Geometry: final body of the model. Coordinates: model frame, mm. Give positions to 0.01 mm unless a question says otherwise; leave off trailing zeros. Write each loop counter-clockwise with the first axis right and the second up, starting at its lowest first coordinate (ties: lowest second). Pieces come first, ordered by that corner, then holes. Notation, with made-up numbers: (61, 77.25) - (90, 77.25) arc R30 ccw to (90, 104.25) - close; hole circle Ø9 at (48, -7). An arc over 180 degrees is marked (long way). Use CSV: the item, a comma, the result in double quotes. Start each with the question number.
(1) Draft query along X for faces 1 (the cylindrical face through (3.44, -167.1, -1.54)), 2 (the flat face through (-155, -506, 1)). Return one class per face: released by +X, released by -X, zero draft, split by the parting line, or undercut.
(2) Section C-C on z = -3.1. Count the separate pieces of the cut face and the enclosed holes in it, and give its area (3 significant figures).
(3) Section A-A on x = -186. Output: boundary loops of the cut face in (y, z), and give its area (3 significant figures).
(4) Section B-B on y = -358. Output: boundary loops of the cut face in (x, z).
(5) Line query: probe 1 along X at (y, z) = (-177.5, 0.25); probe 2 along Y at (x, z) = (-96.5, -1.6); probe 3 along X at (y, z) = (-425, -2.75). Output: solid intervals per line, ascending. Write a range as [from, to].
from build123d import *

# Parameters (mm, degrees)
SKETCH2_W           = 347
SKETCH2_H           = 371
SKETCH2_W_2         = 300
SKETCH2_H_2         = 300
BOSS_EXTRUDE1_DEPTH = 5
SKETCH6_R           = 1.75
CUT_EXTRUDE1_DEPTH  = 10
SKETCH7_W           = 10
SKETCH7_H           = 371
BOSS_EXTRUDE2_DEPTH = 5
SKETCH3_R           = 12
CUT_EXTRUDE2_DEPTH  = 5
SKETCH9_R           = 1.5
CUT_EXTRUDE3_DEPTH  = 6
SKETCH10_R          = 2
CUT_EXTRUDE4_DEPTH  = 5


with BuildPart() as part:
    # Sketch2 → Boss-Extrude1 (new body)
    with BuildSketch(Plane.XY.offset(-4)):
        with Locations((-157.5, -343.5)):
            Rectangle(SKETCH2_W, SKETCH2_H)
        with Locations((-157.5, -350)):
            Rectangle(SKETCH2_W_2, SKETCH2_H_2, mode=Mode.SUBTRACT)
    extrude(amount=BOSS_EXTRUDE1_DEPTH)

    # Sketch6 → Cut-Extrude1 (cut)
    with BuildSketch(Plane(origin=(0, 0, -4), x_dir=(-1, 0, 0), z_dir=(0, 0, -1))):
        with Locations((318.499999962, -490)):
            Circle(SKETCH6_R)
        with Locations((318.499999962, -470)):
            Circle(SKETCH6_R)
        with Locations((318.499999962, -450)):
            Circle(SKETCH6_R)
        with Locations((318.499999962, -430)):
            Circle(SKETCH6_R)
        with Locations((318.499999962, -410)):
            Circle(SKETCH6_R)
        with Locations((318.499999962, -390)):
            Circle(SKETCH6_R)
        with Locations((318.499999962, -370)):
            Circle(SKETCH6_R)
        with Locations((318.499999962, -350)):
            Circle(SKETCH6_R)
        with Locations((318.499999962, -330)):
            Circle(SKETCH6_R)
        with Locations((318.499999962, -310)):
            Circle(SKETCH6_R)
        with Locations((318.499999962, -290)):
            Circle(SKETCH6_R)
        with Locations((318.499999962, -270)):
            Circle(SKETCH6_R)
        with Locations((318.499999962, -250)):
            Circle(SKETCH6_R)
        with Locations((318.499999962, -230)):
            Circle(SKETCH6_R)
        with Locations((318.499999962, -210)):
            Circle(SKETCH6_R)
    cut_extrude1 = extrude(amount=-CUT_EXTRUDE1_DEPTH, mode=Mode.SUBTRACT)

    # Mirror1: Cut-Extrude1 across plane
    add(cut_extrude1.mirror(Plane.ZY.offset(157.5)), mode=Mode.SUBTRACT)

    # Sketch7 → Boss-Extrude2 (add)
    with BuildSketch(Plane.XY.offset(1)):
        with Locations((-336, -343.5)):
            Rectangle(SKETCH7_W, SKETCH7_H)
    boss_extrude2 = extrude(amount=-BOSS_EXTRUDE2_DEPTH)

    # Mirror2: Boss-Extrude2 across plane
    add(boss_extrude2.mirror(Plane.ZY.offset(157.5)))

    # Sketch3 → Cut-Extrude2 (cut)
    with BuildSketch(Plane(origin=(0, 0, -4), x_dir=(-1, 0, 0), z_dir=(0, 0, -1))):
        with Locations((319.999999962, -179)):
            Circle(SKETCH3_R)
    cut_extrude2 = extrude(amount=-CUT_EXTRUDE2_DEPTH, mode=Mode.SUBTRACT)

    # Sketch9 → Cut-Extrude3 (cut, through all)
    with BuildSketch(Plane(origin=(0, 0, -4), x_dir=(-1, 0, 0), z_dir=(0, 0, -1))):
        with Locations((335.266435368, -194.266435406)):
            Circle(SKETCH9_R)
        with Locations((335.266435368, -163.733564594)):
            Circle(SKETCH9_R)
        with Locations((304.733564556, -163.733564594)):
            Circle(SKETCH9_R)
        with Locations((304.733564556, -194.266435406)):
            Circle(SKETCH9_R)
    cut_extrude3 = extrude(amount=-CUT_EXTRUDE3_DEPTH, mode=Mode.SUBTRACT)

    # Mirror3: Cut-Extrude2, Cut-Extrude3 across plane
    add(cut_extrude2.mirror(Plane.ZY.offset(157.5)), mode=Mode.SUBTRACT)
    add(cut_extrude3.mirror(Plane.ZY.offset(157.5)), mode=Mode.SUBTRACT)

    # Sketch10 → Cut-Extrude4 (cut)
    with BuildSketch(Plane.XY.offset(1)):
        with Locations((-319.999999962, -515)):
            Circle(SKETCH10_R)
    cut_extrude4 = extrude(amount=-CUT_EXTRUDE4_DEPTH, mode=Mode.SUBTRACT)

    # Mirror4: Cut-Extrude4 across plane
    add(cut_extrude4.mirror(Plane.ZY.offset(157.5)), mode=Mode.SUBTRACT)


solid = part.part
Check values:
1,face 1,"undercut"
1,face 2,"zero draft"
2,separate pieces,"1"
2,enclosed holes,"43"
2,area,"44,900 mm²"
3,outline,"(-529, -4) - (-500, -4) - (-500, 1) - (-529, 1) - close; (-200, -4) - (-158, -4) - (-158, 1) - (-200, 1) - close"
3,area,"355 mm²"
4,outline,"(-341, -4) - (-307.5, -4) - (-307.5, 1) - (-341, 1) - close; (-7.5, -4) - (26, -4) - (26, 1) - (-7.5, 1) - close"
5,probe 1,"x = [-341, -331.91], [-308.09, -6.91], [16.91, 26]"
5,probe 2,"y = [-529, -500], [-200, -158]"
5,probe 3,"x = [-341, -307.5], [-7.5, 26]"
